from build123d import *

# Parameters (mm, degrees)
SKETCH1_W                = 10
SKETCH1_H                = 10
BOSS_EXTRUDE1_DEPTH      = 5
SKETCH2_W                = 10
SKETCH2_H                = 10
BOSS_EXTRUDE2_DEPTH      = 20
SKETCH3_W                = 60
SKETCH3_H                = 20
SKETCH3_R                = 2
BOSS_EXTRUDE3_DEPTH      = 5
SKETCH4_W                = 10
SKETCH4_H                = 12
BOSS_EXTRUDE4_DEPTH      = 10
BOSS_EXTRUDE4_DEPTH_BACK = 65
SKETCH5_W                = 4.1
SKETCH5_H                = 3.1
SKETCH5_W_2              = 1.6
SKETCH5_H_2              = 2.1
CUT_EXTRUDE1_DEPTH       = 13
SKETCH7_R                = 1
CUT_EXTRUDE3_DEPTH       = 27
SKETCH10_W               = 10
SKETCH10_H               = 10
BOSS_EXTRUDE6_DEPTH      = 10
SKETCH12_W               = 60
SKETCH12_H               = 20
SKETCH12_R               = 2
BOSS_EXTRUDE7_DEPTH      = 5
CHAMFER1_SIZE            = 2


with BuildPart() as part:
    # Sketch1 → Boss-Extrude1 (new body)
    with BuildSketch(Plane.XY):
        Rectangle(SKETCH1_W, SKETCH1_H)
    extrude(amount=BOSS_EXTRUDE1_DEPTH)

    # Sketch2 → Boss-Extrude2 (add)
    with BuildSketch(Plane(origin=(0, 0, 0), x_dir=(-1, 0, 0), z_dir=(0, 0, -1))):
        Rectangle(SKETCH2_W, SKETCH2_H)
    extrude(amount=BOSS_EXTRUDE2_DEPTH)

    # Sketch3 → Boss-Extrude3 (add)
    with BuildSketch(Plane(origin=(0, 0, -20), x_dir=(-1, 0, 0), z_dir=(0, 0, -1))):
        Rectangle(SKETCH3_W, SKETCH3_H)
        with Locations((20, 0)):
            Circle(SKETCH3_R, mode=Mode.SUBTRACT)
        with Locations((-20, 0)):
            Circle(SKETCH3_R, mode=Mode.SUBTRACT)
    extrude(amount=-BOSS_EXTRUDE3_DEPTH)

    # Sketch4 → Boss-Extrude4 (add, two sides)
    with BuildSketch(Plane.XZ.offset(5)) as boss_extrude4_sk:
        Rectangle(SKETCH4_W, SKETCH4_H)
    extrude(amount=BOSS_EXTRUDE4_DEPTH)
    extrude(boss_extrude4_sk.sketch, amount=-BOSS_EXTRUDE4_DEPTH_BACK)

    # Sketch5 → Cut-Extrude1 (cut)
    with BuildSketch(Plane(origin=(0, -15, 0), x_dir=(-1, 0, 0), z_dir=(0, -1, 0))):
        Rectangle(SKETCH5_W, SKETCH5_H)
        with Locations((-2.85, 0)):
            Rectangle(SKETCH5_W_2, SKETCH5_H_2)
    extrude(amount=-CUT_EXTRUDE1_DEPTH, mode=Mode.SUBTRACT)

    # Sketch7 → Cut-Extrude3 (cut, through all)
    with BuildSketch(Plane.XY.offset(6)):
        with Locations((0, -10)):
            Circle(SKETCH7_R)
    extrude(amount=-CUT_EXTRUDE3_DEPTH, mode=Mode.SUBTRACT)

    # Sketch10 → Boss-Extrude6 (add)
    with BuildSketch(Plane(origin=(0, 0, -6), x_dir=(-1, 0, 0), z_dir=(0, 0, -1))):
        with Locations((0, 55)):
            Rectangle(SKETCH10_W, SKETCH10_H)
    extrude(amount=BOSS_EXTRUDE6_DEPTH)

    # Sketch12 → Boss-Extrude7 (add)
    with BuildSketch(Plane(origin=(0, 0, -16), x_dir=(-1, 0, 0), z_dir=(0, 0, -1))):
        with Locations((0, 55)):
            Rectangle(SKETCH12_W, SKETCH12_H)
        with Locations((20, 55)):
            Circle(SKETCH12_R, mode=Mode.SUBTRACT)
        with Locations((-20, 55)):
            Circle(SKETCH12_R, mode=Mode.SUBTRACT)
    extrude(amount=BOSS_EXTRUDE7_DEPTH)

    # Chamfer1
    chamfer1_edges = [part.edges().sort_by_distance(p)[0] for p in [
        (-18, 55, -16),
        (22, 55, -16),
        (-18, 0, -15),
        (22, 0, -15),
    ]]
    chamfer(chamfer1_edges, length=CHAMFER1_SIZE)


solid = part.part
Verification items for the finished model (mm, model axes). A direction names the side the tool comes from. Coordinates: 2 decimals unless noted, no trailing zeros. Write each loop counter-clockwise with the first axis right and the second up, starting at its lowest first coordinate (ties: lowest second). Pieces come first, ordered by that corner, then holes. Notation, with made-up numbers: (56, 81) - (95, 81) arc R23 cw to (95, 107) - close; hole circle Ø10 at (8, 21.25). An arc over 180 degrees is marked (long way). Answer as a JSON object with one key per item and string values.
(1) Mould release check, pull along X, two halves, no side actions. Record for faces 1 (the flat face through (0, -8.6, 1.55)), 2 (the cylindrical face through (20, 57, -19)), 3 (the flat face through (30, 0, -18)), 4 (the flat face through (-2.3, -15, 0.1)): pulls with the +X half, pulls with the -X half, needs draft (parallel to the pull), parting line crosses it, or undercut.
Report:
{"face 1": "undercut", "face 2": "undercut", "face 3": "pulls with the +X half", "face 4": "needs draft"}
(2) Gauge pin test, flat ends, axial feed: pin 1 Ø16 at (x, y) = (-4.5, 2) entering from -Z; pin 2 Ø2.5 at (x, y) = (-20, 0) entering from -Z; pin 3 Ø0.6 at (y, z) = (-9.5, 0) entering from -X; pin 4 Ø2.5 at (x, z) = (-2, -10) entering from +Y. Record the tip position at first contact, or that the pin passes through.
Report:
{"pin 1": "z = -20", "pin 2": "through", "pin 3": "x = -5", "pin 4": "y = 60"}
(3) Cross-section at C-C on x = 0. Give the number of separate pieces and of enclosed holes in the cut face, plus the area to 3 significant figures.
Report:
{"separate pieces": "3", "enclosed holes": "0", "area": "1,230 mm^2"}
(4) Thickness scan on line 1 along Y through (x, z) = (20, -18.95); line 2 along Y through (x, z) = (7, -18.5); line 3 along Y through (x, z) = (0, -2.5). Record the ranges inside material, lowest first.
Report:
{"line 1": "-10 to -2, 2 to 10, 45 to 53, 57 to 65", "line 2": "-10 to 10, 45 to 65", "line 3": "-15 to -11, -9 to 60"}
(5) Cross-section at B-B on y = 55. Record the cut outline in (x, z).
Report:
{"outline": "(-30, -21) - (-22, -21) - (-22, -18) - (-24, -16) - (-30, -16) - close; (-18, -21) - (18, -21) - (18, -18) - (16, -16) - (5, -16) - (5, 6) - (-5, 6) - (-5, -16) - (-16, -16) - (-18, -18) - close; (22, -21) - (30, -21) - (30, -16) - (24, -16) - (22, -18) - close"}
(6) Cross-section at D-D on y = -6. Record the cut outline in (x, z).
Report:
{"outline": "(-30, -20) - (30, -20) - (30, -15) - (-30, -15) - close; (-5, -6) - (5, -6) - (5, 6) - (-5, 6) - close; hole (-2.05, -1.55) - (2.05, -1.55) - (2.05, -1.05) - (3.65, -1.05) - (3.65, 1.05) - (2.05, 1.05) - (2.05, 1.55) - (-2.05, 1.55) - close"}
(7) Tool access check on faces 5 (the flat face through (0, 0, -20)), 6 (the flat face through (0, -5, -10)), 7 (the flat face through (-2.05, -9, 0)). Record the directions out of +Z, -Z, +X, -X, +Y, -Y that give a thin tool (end or side, any length) a straight path to the whole face; none if there is none.
Report:
{"face 5": "-Z, +X, -X, -Y", "face 6": "+X, -X, -Y", "face 7": "-Y"}
(8) Cross-section at A-A on x = 12. Record the cut outline in (y, z), plus the area to 3 significant figures.
Report:
{"outline": "(-10, -20) - (10, -20) - (10, -15) - (-10, -15) - close; (45, -21) - (65, -21) - (65, -16) - (45, -16) - close", "area": "200 mm^2"}
